Autodesk Inventor part; units mm, degrees
ref_plane "YZ Plane" through (0, 0, 0) normal (1, 0, 0) x (0, 1, 0)
ref_plane "XZ Plane" through (0, 0, 0) normal (0, 1, 0) x (-1, 0, 0)
ref_plane "XY Plane" through (0, 0, 0) normal (0, 0, 1) x (1, 0, 0)
sketch "Esquisse1" plane through (0, 0, 0) normal (1, 0, 0) x (0, 1, 0)
  line L0 (35, 45) -> (-35, 45)
  line L1 (-35, 45) -> (-35, -45)
  line L2 (-35, -45) -> (35, -45)
  line L3 (35, -45) -> (35, 45)
  line L4 (26.5459, 0) -> (-33.52, 0) construction
  line L5 (0, 24.5499) -> (0, -29.9835) construction
  point P0 (0, 0)
  dimension "d0" = 90
  dimension "d1" = 70
extrude "Extrusion1" add sketch "Esquisse1" along normal blind 2
sketch "Esquisse2" plane through (2, 0, 0) normal (1, 0, 0) x (0, 0, -1)
  line L0 (-43, 33) -> (43, 33)
  line L1 (43, 33) -> (43, -33)
  line L2 (43, -33) -> (-43, -33)
  line L3 (-43, -33) -> (-43, 33)
  line L4 (-41, 31) -> (41, 31)
  line L5 (41, 31) -> (41, -31)
  line L6 (41, -31) -> (-41, -31)
  line L7 (-41, -31) -> (-41, 31)
  line L8 (45, 35) -> (-45, 35)
  line L9 (-45, 35) -> (-45, -35)
  line L10 (-45, -35) -> (45, -35)
  line L11 (45, -35) -> (45, 35)
  dimension "d4" = 2
  dimension "d5" = 2
  dimension "d6" = 2
  dimension "d7" = 2
  dimension "d8" = 2
  dimension "d9" = 2
  dimension "d10" = 2
  dimension "d11" = 2
extrude "Extrusion2" add sketch "Esquisse2" along normal blind 8 contours L0 L1 L2 L3
sketch "Esquisse3" plane through (0, -35, -45) normal (0, 0, -1) x (-1, 0, 0)
  point P0 (0, 35)
sketch "Esquisse4" plane through (2, 0, 0) normal (1, 0, 0) x (0, 0, -1)
  line L0 (45, -35) -> (45, 35)
  line L1 (45, -7.5) -> (52, -7.5)
  line L2 (52, -7.5) -> (52, 7.5)
  line L3 (52, 7.5) -> (45, 7.5)
  line L4 (45, 7.5) -> (45, -7.5)
  point P0 (0, 0)
  dimension "d14" = 15
  dimension "d15" = 7
  dimension "d16" = 27.5
extrude "Extrusion3" add sketch "Esquisse4" against normal blind 2
fillet "Congé1" radius 2 5 edges at (1, 35, -45) (1, 7.5, -52) (1, -7.5, -52) (1, 7.5, -45) (1, -35, -45)
fillet "Congé2" radius 2 1 edges at (1, -7.5, -45)
mirror "Mise en miroir1" about plane through (0, 0, 0) normal (0, 0, 1) of "Extrusion3"
fillet "Congé3" radius 2 5 edges at (1, -35, 45) (1, -7.5, 45) (1, -7.5, 52) (1, 7.5, 52) (1, 35, 45)
fillet "Congé4" radius 2 1 edges at (1, 7.5, 45)
sketch "Esquisse5" plane through (0, 0, 0) normal (-1, 0, 0) x (0, 0, 1)
  circle A0 centre (-48, 3.5) radius 1.75
  line L0 (-52, 5.5) -> (-52, -5.5)
  line L1 (-47, 7.5) -> (-50, 7.5)
  point P0 (0, 0)
  dimension "d23" = 3.5
  dimension "d24" = 4
  dimension "d25" = 4
extrude "Extrusion4" cut sketch "Esquisse5" against normal blind 2
mirror "Mise en miroir2" about plane through (0, 0, 0) normal (0, 1, 0) of "Extrusion4"
mirror "Mise en miroir3" about plane through (0, 0, 0) normal (0, 0, 1) of "Extrusion4", "Mise en miroir2"
properties part number "Couv"
Model file for the job. Use its own axes, mm. A direction names the side the tool comes from. Coordinates: 2 decimals unless noted, no trailing zeros. Write each loop counter-clockwise with the first axis right and the second up, starting at its lowest first coordinate (ties: lowest second). Pieces come first, ordered by that corner, then holes. Notation, with made-up numbers: (53.5, 89.25) - (104.5, 89.25) arc R17 cw to (104.5, 105.25) - close; hole circle Ø3 at (16.5, 26). An arc over 180 degrees is marked (long way). Use a Markdown table: item, result. Add a question column.
Item 1: Drop flat-ended pins along their axis: pin 1 (4 mm diameter, centred on x = 5, z = 4.5, fed in from -Y); pin 2 (2 mm diameter, centred on y = -3.5, z = -48, fed in from -X); pin 3 (3 mm diameter, centred on x = 7, y = 4, fed in from -Z); pin 4 (2 mm diameter, centred on x = 1.5, z = -48, fed in from +Y). Give the stop position or say it passes through.
Item 2: Band-saw the part on D-D, the plane y = 15. Write the cut outline in (x, z), and give its area (3 significant figures).
Item 3: Two-plate mould, pull along Z, no slides. Class faces 6 (the face through (0.99, -6.93, 51.4)), 7 (the face through (6, 0, -41)), 8 (the face through (1.01, 34.4, -44.43)): pulls with the +Z half, pulls with the -Z half, needs draft (parallel to the pull), parting line crosses it, or undercut.
Item 4: 3-axis set-ups, long thin cutter, end or side, ignore diameter. For faces 1 (the face through (6, 33, 1)), 2 (the face through (1, 7.5, -49)), 3 (the face through (1, 7.5, 48)), 4 (the face through (1, -21, 45)), 5 (the face through (1, -21, -45)): which of +Z, -Z, +X, -X, +Y, -Y reach the whole face in a straight line?
Item 5: Band-saw the part on B-B, the plane x = 7.75. Write the cut outline in (y, z), and give its area (3 significant figures).
Item 6: Drill centre lines: line 1 along Y through (x, z) = (1.25, -48); line 2 along Y through (x, z) = (5.25, -33); line 3 along Z through (x, y) = (4, -26.5). Where is each one in solid material? Low to high.
Item 7: Band-saw the part on A-A, the plane y = -3.5. Write the cut outline in (x, z), and give its area (3 significant figures).
Item 8: Band-saw the part on C-C, the plane z = -5.5. Write the cut outline in (x, y).
A:
| question | item | result |
|---|---|---|
| 1 | pin 1 | stops at y = -33 |
| 1 | pin 2 | passes through |
| 1 | pin 3 | stops at z = -43 |
| 1 | pin 4 | stops at y = 7.5 |
| 2 | outline | (0, -45) - (2, -45) - (2, -43) - (10, -43) - (10, -41) - (2, -41) - (2, 41) - (10, 41) - (10, 43) - (2, 43) - (2, 45) - (0, 45) - close |
| 2 | area | 212 mm² |
| 3 | face 6 | pulls with the +Z half |
| 3 | face 7 | undercut |
| 3 | face 8 | pulls with the -Z half |
| 4 | face 1 | +Z, -Z, +X, +Y |
| 4 | face 2 | -Z, +X, -X, +Y |
| 4 | face 3 | +Z, +X, -X, +Y |
| 4 | face 4 | +Z, +X, -X, -Y |
| 4 | face 5 | -Z, +X, -X, -Y |
| 5 | outline | (-33, -43) - (33, -43) - (33, 43) - (-33, 43) - close; hole (-31, -41) - (31, -41) - (31, 41) - (-31, 41) - close |
| 5 | area | 592 mm² |
| 6 | line 1 | y = -7.5 to -5.25, -1.75 to 1.75, 5.25 to 7.5 |
| 6 | line 2 | y = -33 to -31, 31 to 33 |
| 6 | line 3 | z = -43 to -41, 41 to 43 |
| 7 | outline | (0, -52) - (2, -52) - (2, -49.75) - (0, -49.75) - close; (0, -46.25) - (2, -46.25) - (2, -43) - (10, -43) - (10, -41) - (2, -41) - (2, 41) - (10, 41) - (10, 43) - (2, 43) - (2, 46.25) - (0, 46.25) - close; (0, 49.75) - (2, 49.75) - (2, 52) - (0, 52) - close |
| 7 | area | 226 mm² |
| 8 | outline | (0, -35) - (2, -35) - (2, -33) - (10, -33) - (10, -31) - (2, -31) - (2, 31) - (10, 31) - (10, 33) - (2, 33) - (2, 35) - (0, 35) - close |
